Input: part model. Units: mm. Frame: model coordinates. A direction names the side the tool comes from. Give positions to 0.01 mm unless a question says otherwise; leave off trailing zeros. Loops run counter-clockwise (first coordinate to the right, second up) from the corner with the lowest first, then second, coordinate; pieces in that order, holes last. Notation, with made-up numbers: (45, 49) - (103, 49) arc R25 ccw to (103, 79) - close; hole circle Ø11 at (82, 81). An arc over 180 degrees is marked (long way). One line per question, with ' | ' between items. Start each with the question number.
from build123d import *

# Parameters (mm, degrees)
SKETCH1_W           = 127
SKETCH1_H           = 91.44
BOSS_EXTRUDE1_DEPTH = 228.6
SKETCH3_W           = 120.65
SKETCH3_H           = 85.09
CUT_EXTRUDE1_DEPTH  = 226.06
SKETCH2_R           = 2.667
CUT_EXTRUDE2_DEPTH  = 266.475570251
SKETCH4_R           = 1.143
BOSS_EXTRUDE3_DEPTH = 5.08
SKETCH5_R           = 20.32
CUT_EXTRUDE3_DEPTH  = 1.27
FILLET1_R           = 0.762
FILLET2_R           = 0.762
FILLET3_R           = 0.762
SKETCH6_W           = 60.96
SKETCH6_H           = 25.4
CUT_EXTRUDE4_DEPTH  = 256.582569828
FILLET4_R           = 2.54
SKETCH7_W           = 85.09
SKETCH7_H           = 111.152565629
CUT_EXTRUDE5_DEPTH  = 268.942913323
SKETCH10_R          = 2.667
CUT_EXTRUDE6_DEPTH  = 2.54
CUT_EXTRUDE7_DEPTH  = 7.62
SKETCH13_R          = 2.667
CUT_EXTRUDE8_DEPTH  = 2.54
CUT_EXTRUDE9_DEPTH  = 7.62


with BuildPart() as part:
    # Sketch1 → Boss-Extrude1 (new body)
    with BuildSketch(Plane(origin=(0, 0, 0), x_dir=(1, 0, 0), z_dir=(0, 1, 0))):
        Rectangle(SKETCH1_W, SKETCH1_H)
    extrude(amount=BOSS_EXTRUDE1_DEPTH)

    # Sketch3 → Cut-Extrude1 (cut)
    with BuildSketch(Plane.XZ):
        Rectangle(SKETCH3_W, SKETCH3_H)
    extrude(amount=-CUT_EXTRUDE1_DEPTH, mode=Mode.SUBTRACT)

    # Sketch2 → Cut-Extrude2 (cut, through all)
    with BuildSketch(Plane(origin=(63.5, 0, 0), x_dir=(0, 0, -1), z_dir=(1, 0, 0))):
        with Locations((0, 182.88)):
            Circle(SKETCH2_R)
    extrude(amount=-CUT_EXTRUDE2_DEPTH, mode=Mode.SUBTRACT)

    # Sketch4 → Boss-Extrude3 (add)
    with BuildSketch(Plane(origin=(63.5, 0, 0), x_dir=(0, 0, -1), z_dir=(1, 0, 0))):
        with Locations(Location((-40.64, 223.52, 0), (0, 0, 180))):
            Circle(SKETCH4_R)
        with Locations(Location((40.64, 223.52, 0), (0, 0, 180))):
            Circle(SKETCH4_R)
        with Locations(Location((40.64, 142.24, 0), (0, 0, 180))):
            Circle(SKETCH4_R)
        with Locations(Location((-40.64, 142.24, 0), (0, 0, 180))):
            Circle(SKETCH4_R)
    boss_extrude3 = extrude(amount=BOSS_EXTRUDE3_DEPTH)

    # Sketch5 → Cut-Extrude3 (cut)
    with BuildSketch(Plane.ZY.offset(-60.325)):
        with Locations((0, 182.88)):
            Circle(SKETCH5_R)
    cut_extrude3 = extrude(amount=-CUT_EXTRUDE3_DEPTH, mode=Mode.SUBTRACT)

    # Fillet1
    fillet1_edges = [part.edges().sort_by_distance(p)[0] for p in [
        (61.595, 182.88, 2.667),
    ]]
    fillet(fillet1_edges, radius=FILLET1_R)

    # Fillet2
    fillet2_edges = [part.edges().sort_by_distance(p)[0] for p in [
        (63.5, 182.88, 2.667),
    ]]
    fillet(fillet2_edges, radius=FILLET2_R)

    # Mirror2: Boss-Extrude3, Cut-Extrude3 across plane
    add(boss_extrude3.mirror(Plane(origin=(0, 0, 0), x_dir=(0, 0, 1), z_dir=(1, 0, 0))))
    add(cut_extrude3.mirror(Plane(origin=(0, 0, 0), x_dir=(0, 0, 1), z_dir=(1, 0, 0))), mode=Mode.SUBTRACT)

    # Fillet3
    fillet3_edges = [part.edges().sort_by_distance(p)[0] for p in [
        (-63.5, 182.88, 2.667),
        (-61.595, 182.88, 2.667),
    ]]
    fillet(fillet3_edges, radius=FILLET3_R)

    # Sketch6 → Cut-Extrude4 (cut, through all)
    with BuildSketch(Plane.XY.offset(45.72)):
        with Locations((0, 182.88)):
            Rectangle(SKETCH6_W, SKETCH6_H)
    extrude(amount=-CUT_EXTRUDE4_DEPTH, mode=Mode.SUBTRACT)

    # Fillet4
    fillet4_edges = [part.edges().sort_by_distance(p)[0] for p in [
        (-63.5, 228.6, 0),
        (0, 228.6, 45.72),
        (63.5, 228.6, 0),
        (63.5, 114.3, 45.72),
        (-63.5, 114.3, 45.72),
        (-63.5, 114.3, -45.72),
        (63.5, 114.3, -45.72),
        (0, 228.6, -45.72),
    ]]
    fillet(fillet4_edges, radius=FILLET4_R)

    # Sketch7 → Cut-Extrude5 (cut, through all)
    with BuildSketch(Plane(origin=(63.5, 0, 0), x_dir=(0, 0, -1), z_dir=(1, 0, 0))):
        with Locations((0, 75.896282814)):
            Rectangle(SKETCH7_W, SKETCH7_H)
    extrude(amount=-CUT_EXTRUDE5_DEPTH, mode=Mode.SUBTRACT)

    # Sketch10 → Cut-Extrude6 (cut)
    with BuildSketch(Plane.ZY.offset(-60.325)):
        with Locations((-30.48, 182.88)):
            Circle(SKETCH10_R)
    extrude(amount=-CUT_EXTRUDE6_DEPTH, mode=Mode.SUBTRACT)

    # Sketch12 → Cut-Extrude7 (cut)
    with BuildSketch(Plane(origin=(0, 0, -45.72), x_dir=(-1, 0, 0), z_dir=(0, 0, -1))):
        Polygon((-34.810362372, 182.807903476), (-34.810362372, 200.587903476), (-60.210362372, 200.587903476), (-60.210362372, 182.807903476), (-60.210362372, 165.027903476), (-34.810362372, 165.027903476), align=None)
    extrude(amount=-CUT_EXTRUDE7_DEPTH, mode=Mode.SUBTRACT)

    # Sketch13 → Cut-Extrude8 (cut)
    with BuildSketch(Plane(origin=(-60.325, 0, 0), x_dir=(0, 0, -1), z_dir=(1, 0, 0))):
        with Locations((-30.48, 182.88)):
            Circle(SKETCH13_R)
    extrude(amount=-CUT_EXTRUDE8_DEPTH, mode=Mode.SUBTRACT)

    # Sketch16 → Cut-Extrude9 (cut)
    with BuildSketch(Plane.XY.offset(45.72)):
        Polygon((-60.34639287, 182.934228321), (-60.34639287, 200.714228321), (-34.94639287, 200.714228321), (-34.94639287, 165.154228321), (-60.34639287, 165.154228321), align=None)
    extrude(amount=-CUT_EXTRUDE9_DEPTH, mode=Mode.SUBTRACT)


solid = part.part
Q1. First-contact query: pin 1 (1 mm diameter, centred on x = 61.5, z = 4.5, fed in from -Y); pin 2 (6 mm diameter, centred on x = -9, z = -13, fed in from -Y); pin 3 (3.5 mm diameter, centred on y = 190, z = -45, fed in from +X); pin 4 (1 mm diameter, centred on y = 185.5, z = 44.5, fed in from -X). Flat tips, straight axial feed; report the tip coordinate or a pass-through.
Q2. Access query for faces 1 (the face through (-47, 165.154, 44)), 2 (the face through (-61.595, 179, 0)), 3 (the face through (60.325, 10, -1)). Directions: +Z, -Z, +X, -X, +Y, -Y. A direction counts if a zero-diameter tool reaches every point of the face in a straight line with its end or side. Return the directions, or none.
Q3. Section B-B, the plane y = 24. Output: boundary loops of the cut face in (x, z) (3 decimals).
Q4. Section C-C, the plane z = 30.48. Output: boundary loops of the cut face in (x, y) (3 decimals), plus the area to 3 significant figures.
Q5. Section D-D, the plane y = 211. Output: boundary loops of the cut face in (x, z) (3 decimals).
Q6. Section A-A, the plane x = 56. Output: boundary loops of the cut face in (y, z) (3 decimals).
Q7. Draft query along Y for faces 4 (the face through (-5, 0, 44)), 5 (the face through (-60.325, 10, -1)), 6 (the face through (-62.54, 184.68, 1.97)). Return one class per face: +Y half, -Y half, draft (parallel to the pull), parting line (faces both ways), or undercut.
Q8. Line query: L1, parallel to Y at x = -61.25, z = 0; L2, parallel to Y at x = -61, z = 30; L3, parallel to Z at x = 32.5, y = 154.5 (3 decimals). Output: solid intervals per line, ascending. Write a range as from..to.
Solved:
1) pin 1: stops at y = 0 | pin 2: stops at y = 226.06 | pin 3: stops at x = 63.5 | pin 4: stops at x = -63.36
2) face 1: +Z | face 2: none | face 3: -Y
3) outline: (-63.5, -43.18) arc R2.54 ccw to (-60.96, -45.72) - (60.96, -45.72) arc R2.54 ccw to (63.5, -43.18) - (63.5, -42.545) - (-63.5, -42.545) - close; (-63.5, 42.545) - (63.5, 42.545) - (63.5, 43.18) arc R2.54 ccw to (60.96, 45.72) - (-60.96, 45.72) arc R2.54 ccw to (-63.5, 43.18) - close
4) outline: (-63.5, 0) - (-60.325, 0) - (-60.325, 20.32) - (-63.5, 20.32) - close; (-63.5, 131.473) - (-60.325, 131.473) - (-60.325, 180.213) - (-62.865, 180.213) - (-62.865, 185.547) - (-60.325, 185.547) - (-60.325, 226.06) - (60.325, 226.06) - (60.325, 131.473) - (63.5, 131.473) - (63.5, 226.06) arc R2.54 ccw to (60.96, 228.6) - (-60.96, 228.6) arc R2.54 ccw to (-63.5, 226.06) - close; (60.325, 0) - (63.5, 0) - (63.5, 20.32) - (60.325, 20.32) - close | area: 1,040 mm²
5) outline: (-63.5, -43.18) arc R2.54 ccw to (-60.96, -45.72) - (60.96, -45.72) arc R2.54 ccw to (63.5, -43.18) - (63.5, 43.18) arc R2.54 ccw to (60.96, 45.72) - (-60.96, 45.72) arc R2.54 ccw to (-63.5, 43.18) - close; hole (-60.325, -42.545) - (60.325, -42.545) - (60.325, 42.545) - (-60.325, 42.545) - close
6) outline: (0, -45.72) - (165.028, -45.72) - (165.028, -42.545) - (0, -42.545) - close; (0, 42.545) - (226.06, 42.545) - (226.06, -42.545) - (200.588, -42.545) - (200.588, -45.72) - (226.06, -45.72) arc R2.54 ccw to (228.6, -43.18) - (228.6, 43.18) arc R2.54 ccw to (226.06, 45.72) - (0, 45.72) - close
7) face 4: -Y half | face 5: draft | face 6: undercut
8) L1: y = 0..20.32, 131.47..162.56, 203.2..228.58 | L2: y = 0..20.32, 131.47..180.26, 185.5..228.6 | L3: z = -45.72..-42.545, 42.545..45.72
